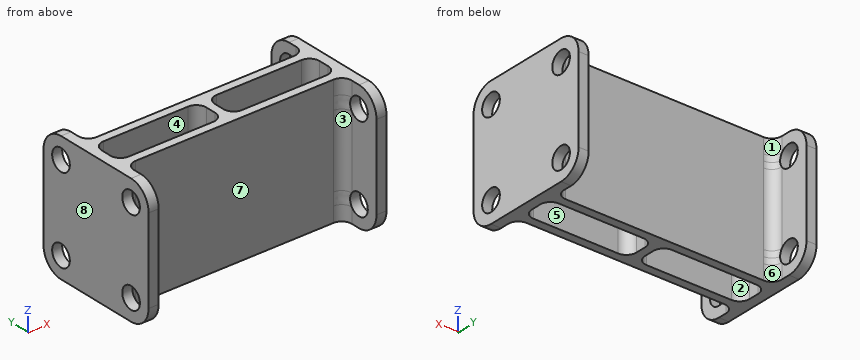
from build123d import *

# Parameters (mm, degrees)
SKETCH_W     = 31.23
SKETCH_H     = 9.12
PAD_DEPTH    = 38.1
SKETCH001_R  = 3.2
POCKET_DEPTH = 71
FILLET_R     = 6.35
FILLET001_R  = 3


with BuildPart() as part:
    # Sketch → Pad (new body)
    with BuildSketch(Plane.XY):
        Polygon((-32.5, 7.1), (32.5, 7.1), (32.5, 19.05), (35.5, 19.05), (35.5, -19.05), (32.5, -19.05), (32.5, -7.1), (-32.5, -7.1), (-32.5, -19.05), (-35.5, -19.05), (-35.5, 19.05), (-32.5, 19.05), align=None)
        with Locations((16.885, 0)):
            Rectangle(SKETCH_W, SKETCH_H, mode=Mode.SUBTRACT)
        with Locations((-16.885, 0)):
            Rectangle(SKETCH_W, SKETCH_H, mode=Mode.SUBTRACT)
    extrude(amount=PAD_DEPTH)

    # Sketch001 (on Face10 of Pad) → Pocket (cut)
    with BuildSketch(Plane(origin=(-35.5, 0, 0), x_dir=(0, -1, 0), z_dir=(-1, 0, 0))):
        with Locations((12.7, 31.75)):
            Circle(SKETCH001_R)
        with Locations((12.7, 6.35)):
            Circle(SKETCH001_R)
        with Locations((-12.7, 6.35)):
            Circle(SKETCH001_R)
        with Locations((-12.7, 31.75)):
            Circle(SKETCH001_R)
    extrude(amount=-POCKET_DEPTH, mode=Mode.SUBTRACT)

    # Fillet
    fillet_edges = [part.edges().sort_by_distance(p)[0] for p in [
        (-34, 19.05, 0),
        (-34, -19.05, 0),
        (34, -19.05, 38.1),
        (34, 19.05, 0),
        (34, -19.05, 0),
        (34, 19.05, 38.1),
        (-34, 19.05, 38.1),
        (-34, -19.05, 38.1),
    ]]
    fillet(fillet_edges, radius=FILLET_R)

    # Fillet001
    fillet001_edges = [part.edges().sort_by_distance(p)[0] for p in [
        (-1.27, -4.56, 19.05),
        (-1.27, 4.56, 19.05),
        (32.5, 4.56, 19.05),
        (32.5, -4.56, 19.05),
        (1.27, -4.56, 19.05),
        (1.27, 4.56, 19.05),
        (-32.5, -4.56, 19.05),
        (-32.5, 4.56, 19.05),
        (-32.5, -7.1, 19.05),
        (-32.5, 7.1, 19.05),
        (32.5, 7.1, 19.05),
        (32.5, -7.1, 19.05),
    ]]
    fillet(fillet001_edges, radius=FILLET001_R)


solid = part.part
Read the model definition and answer for the solid it produces. Units are mm, in the model's axes. Face numbers are marked on the shaded views. A direction names the side the tool comes from. Give positions to 0.01 mm unless a question says otherwise; leave off trailing zeros. Loops run counter-clockwise (first coordinate to the right, second up) from the corner with the lowest first, then second, coordinate; pieces in that order, holes last. Notation, with made-up numbers: M 26,-26.5 L 79,-26.5 A25 cw 79,7.5 Z; hole C -38.75,6.5 d1. An arc over 180 degrees is marked long. Write each question's results on one line, items separated by ' | '.
1. Straight lines are drawn through the part: line 1 (X direction, y = 17, z = 25.5); line 2 (Y direction, x = -22, z = 26); line 3 (Z direction, x = 33, y = -12). For each, find the intervals that lie inside material, in ascending order. Write a range as [from, to].
Values:
line 1: x = [-35.5, -32.5], [32.5, 35.5] | line 2: y = [-7.1, -4.56], [4.56, 7.1] | line 3: z = [0, 3.23], [9.47, 28.63], [34.87, 38.1]
2. Section B-B on z = 16 is taken. State how many separate pieces and enclosed holes the cut face has, plus the area to 3 significant figures.
Values:
separate pieces: 1 | enclosed holes: 2 | area: 605 mm^2
3. Section C-C on y = 17.5 is taken. Give the vertices of the cut face in (x, z), plus the area to 3 significant figures.
Values:
outline: M -35.5,2.19 L -32.5,2.19 L -32.5,35.91 L -35.5,35.91 Z; M 32.5,2.19 L 35.5,2.19 L 35.5,35.91 L 32.5,35.91 Z | area: 202 mm^2
4. Given pin 1 (7.5 mm diameter, centred on x = -20, z = 19.5, fed in from +Y); pin 2 (5 mm diameter, centred on y = 12.7, z = 6.35, fed in from -X); pin 3 (7.5 mm diameter, centred on x = 19.5, z = 20.5, fed in from -Y), each flat-ended and moving along its own axis, determine where each tip first touches the part or whether it passes through.
Values:
pin 1: stops at y = 7.1 | pin 2: passes through | pin 3: stops at y = -7.1
5. A tool of negligible diameter and unlimited length cuts with its end or side. For the marked faces 5, 6, 7 and 8, from which of +Z, -Z, +X, -X, +Y, -Y can it reach the whole face along a straight path? Write none if from no direction.
Values:
face 5: +Z, -Z | face 6: +Z, -Z, +Y | face 7: +Z, -Z, -Y | face 8: +Z, -Z, -X, +Y, -Y
6. The mould has two halves that part along Y. Classify the marked faces 1, 2, 3 and 4: pulls with the +Y half, pulls with the -Y half, needs draft (parallel to the pull), parting line crosses it, or undercut.
Values:
face 1: pulls with the +Y half | face 2: undercut | face 3: pulls with the -Y half | face 4: undercut
7. Section A-A on x = -11 is taken. Give the vertices of the cut face in (y, z), plus the area to 3 significant figures.
Values:
outline: M -7.1,0 L -4.56,0 L -4.56,38.1 L -7.1,38.1 Z; M 4.56,0 L 7.1,0 L 7.1,38.1 L 4.56,38.1 Z | area: 194 mm^2
